from build123d import *

# Parameters (mm, degrees)
SKETCH1_W           = 19.05
SKETCH1_H           = 6.35
SKETCH1_W_2         = 12.7
SKETCH1_H_2         = 38.1
BOSS_EXTRUDE1_DEPTH = 25.4
CUT_EXTRUDE1_REACH  = 8.35
SKETCH2_R           = 3.175
CUT_EXTRUDE2_REACH  = 33.75
SKETCH3_R           = 2
CUT_EXTRUDE3_REACH  = 33.75
SKETCH4_W           = 25.4
SKETCH4_H           = 13.240999966


with BuildPart() as part:
    # Sketch1 → Boss-Extrude1 (new body)
    with BuildSketch(Plane.XY):
        with Locations((-15.875, -15.875)):
            Rectangle(SKETCH1_W, SKETCH1_H)
        Rectangle(SKETCH1_W_2, SKETCH1_H_2)
    extrude(amount=BOSS_EXTRUDE1_DEPTH)

    # Sketch2 → Cut-Extrude1 (cut, up to next)
    with BuildSketch(Plane(origin=(0, -12.7, 0), x_dir=(1, 0, 0), z_dir=(0, 1, 0)), mode=Mode.PRIVATE) as cut_extrude1_sk1:
        with Locations((-15.875, -6.35)):
            Circle(SKETCH2_R)
    cut_extrude1_tool1 = extrude(cut_extrude1_sk1.sketch, amount=-CUT_EXTRUDE1_REACH, mode=Mode.PRIVATE) & part.part
    add(cut_extrude1_tool1.solids().sort_by_distance((-15.875, -12.7, 6.35))[0], mode=Mode.SUBTRACT)
    # Sketch2 → Cut-Extrude1 (cut, up to next)
    with BuildSketch(Plane(origin=(0, -12.7, 0), x_dir=(1, 0, 0), z_dir=(0, 1, 0)), mode=Mode.PRIVATE) as cut_extrude1_sk2:
        with Locations((-15.875, -19.05)):
            Circle(SKETCH2_R)
    cut_extrude1_tool2 = extrude(cut_extrude1_sk2.sketch, amount=-CUT_EXTRUDE1_REACH, mode=Mode.PRIVATE) & part.part
    add(cut_extrude1_tool2.solids().sort_by_distance((-15.875, -12.7, 19.05))[0], mode=Mode.SUBTRACT)

    # Sketch3 → Cut-Extrude2 (cut, up to next)
    with BuildSketch(Plane(origin=(6.35, 0, 0), x_dir=(0, 0, -1), z_dir=(1, 0, 0)), mode=Mode.PRIVATE) as cut_extrude2_sk1:
        with Locations((-12.7, -1.810999966)):
            Circle(SKETCH3_R)
    cut_extrude2_tool1 = extrude(cut_extrude2_sk1.sketch, amount=-CUT_EXTRUDE2_REACH, mode=Mode.PRIVATE) & part.part
    add(cut_extrude2_tool1.solids().sort_by_distance((6.35, -1.811, 12.7))[0], mode=Mode.SUBTRACT)

    # Sketch4 → Cut-Extrude3 (cut, up to next)
    with BuildSketch(Plane(origin=(6.35, 0, 0), x_dir=(0, 0, -1), z_dir=(1, 0, 0)), mode=Mode.PRIVATE) as cut_extrude3_sk1:
        with Locations((-12.7, 12.429500017)):
            Rectangle(SKETCH4_W, SKETCH4_H)
    cut_extrude3_tool1 = extrude(cut_extrude3_sk1.sketch, amount=-CUT_EXTRUDE3_REACH, mode=Mode.PRIVATE) & part.part
    add(cut_extrude3_tool1.solids().sort_by_distance((6.35, 12.4295, 12.7))[0], mode=Mode.SUBTRACT)


solid = part.part
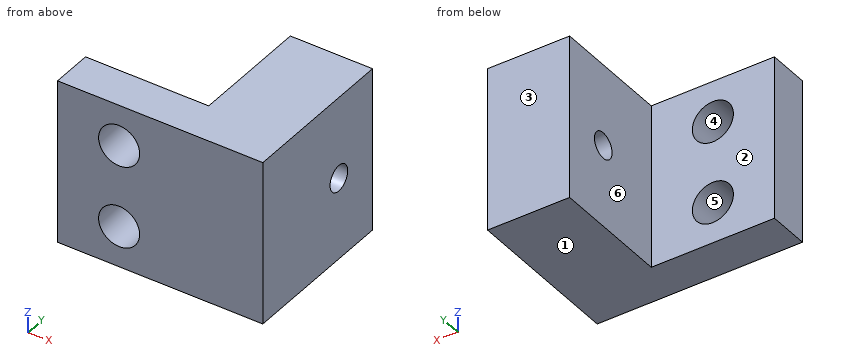
Could you check a few things on this model? Use its own coordinates, in mm. Face numbers are marked on the shaded views. A direction names the side the tool comes from. Give positions to 0.01 mm unless a question says otherwise; leave off trailing zeros. Write each loop counter-clockwise with the first axis right and the second up, starting at its lowest first coordinate (ties: lowest second). Pieces come first, ordered by that corner, then holes. Notation, with made-up numbers: (71, 46) - (125, 46) arc R27 ccw to (125, 66) - close; hole circle Ø7 at (18.25, 43). An arc over 180 degrees is marked (long way). Use CSV: the item, a comma, the result in double quotes. Start each with the question number.
Item 1: I'm going to push flat-ended pins straight in: pin 1 (7.5 mm diameter, centred on x = -15.875, z = 6.35, fed in from +Y); pin 2 (5.5 mm diameter, centred on x = -15.875, z = 19.05, fed in from +Y). Where does each tip first touch, or does it pass through?
Item 2: If we mould it in two halves opening along X, with no side actions, what happens to the marked faces 3, 4, 5 and 6? For each: pulls with the +X half, pulls with the -X half, needs draft (parallel to the pull), parting line crosses it, or undercut.
Item 3: I want a section at B-B, the plane x = -17. Please give me the cut outline in (y, z).
Item 4: If I drill on line 1 along X through (y, z) = (-12.75, 19); line 2 along Y through (x, z) = (1.25, 12.7); line 3 along X through (y, z) = (-5.5, 21.5), over which ranges is the centre line in solid material (lowest first)?
Item 5: I want a section at A-A, the plane z = 19.05. Please give me the cut outline in (x, y).
Item 6: I want a section at C-C, the plane y = -3. Please give me the cut outline in (x, z), then the cut area to 3 significant figures.
Item 7: I want a section at D-D, the plane y = -14.5. Please give me the cut outline in (x, z) (3 decimals).
Item 8: For the marked faces 1 and 2, which set-ups out of +Z, -Z, +X, -X, +Y, -Y let a thin tool reach every point of the face, with its end or its side?
Findings:
1,pin 1,"stops at y = -12.7"
1,pin 2,"passes through"
2,face 3,"needs draft"
2,face 4,"undercut"
2,face 5,"undercut"
2,face 6,"pulls with the -X half"
3,outline,"(-19.05, 0) - (-12.7, 0) - (-12.7, 3.38) - (-19.05, 3.38) - close; (-19.05, 9.32) - (-12.7, 9.32) - (-12.7, 16.08) - (-19.05, 16.08) - close; (-19.05, 22.02) - (-12.7, 22.02) - (-12.7, 25.4) - (-19.05, 25.4) - close"
4,line 1,"x = -25.4 to -19.05, -12.7 to 6.35"
4,line 2,"y = -19.05 to -3.81, 0.19 to 5.81"
4,line 3,"x = -6.35 to 6.35"
5,outline,"(-25.4, -19.05) - (-19.05, -19.05) - (-19.05, -12.7) - (-25.4, -12.7) - close; (-12.7, -19.05) - (6.35, -19.05) - (6.35, 5.81) - (-6.35, 5.81) - (-6.35, -12.7) - (-12.7, -12.7) - close"
6,outline,"(-6.35, 0) - (6.35, 0) - (6.35, 11.09) - (-6.35, 11.09) - close; (-6.35, 14.31) - (6.35, 14.31) - (6.35, 25.4) - (-6.35, 25.4) - close"
6,area,"282 mm2"
7,outline,"(-25.4, 0) - (6.35, 0) - (6.35, 25.4) - (-25.4, 25.4) - close; hole circle Ø6.35 at (-15.875, 6.35); hole circle Ø6.35 at (-15.875, 19.05)"
8,face 1,"-Z, +X, -X, +Y, -Y"
8,face 2,"+Z, -Z, -X, +Y"
